The listing builds one solid part. Answer for the finished solid, in the listing's coordinates (mm). A direction names the side the tool comes from. Give positions to 0.01 mm unless a question says otherwise; leave off trailing zeros. Loops run counter-clockwise (first coordinate to the right, second up) from the corner with the lowest first, then second, coordinate; pieces in that order, holes last. Notation, with made-up numbers: M 77,-25.75 L 122,-25.75 A22 cw 122,-15.75 Z; hole C 86.25,50 d10. An arc over 180 degrees is marked long. One line per item, written item: value. Start each with the question number.
Q1. For faces 1 (the flat face through (-2, -1.4, 1.3)), 2 (the conical face through (-0.09, -1.44, 2.52)), determine the directions among +Z, -Z, +X, -X, +Y, -Y from which every point of the face is accessible in a straight line to the end or side of a thin tool.
Q2. A cutting plane is placed at A-A, the plane x = -11.5. Determine the outline of the cut face in (y, z), and give its area (3 significant figures).
Q3. Consider L1, parallel to X at y = 0.5, z = -2.3; L2, parallel to Y at x = -5, z = -0.6; L3, parallel to Y at x = -13, z = -0.8. Determine where each line is inside the solid, lowest interval first.
Q4. Flat-ended cylindrical pins translate along their axes: pin 1 (1.5 mm diameter, centred on x = -29.5, y = 2, fed in from -Z); pin 2 (2 mm diameter, centred on x = -9.5, z = 1.5, fed in from -Y); pin 3 (1.6 mm diameter, centred on y = -1, z = 0.5, fed in from -X); pin 4 (1 mm diameter, centred on y = -1, z = 2, fed in from -X). Find the tip coordinate at first contact, or state that the pin passes through.
from build123d import *

# Parameters (mm, degrees)
DODANIE_WYCI_GNI_CIE1_DEPTH = 2
SFAZOWANIE1_SIZE            = 0.5


with BuildPart() as part:
    # Szkic1 → Obrót1 (revolve)
    with BuildSketch(Plane.XY):
        Polygon((0, 0), (0, 2.75), (-2, 2.75), (-2, 1.5), (-37, 1.5), (-37, 0), align=None)
    revolve(axis=Axis((-37, 0, 0), (1, 0, 0)))

    # Szkic2 → Dodanie-wyciągnięcie1 (add)
    with BuildSketch(Plane(origin=(0, 0, 0), x_dir=(0, 0, -1), z_dir=(1, 0, 0))):
        Polygon((-2.75, 1.58771324), (-2.75, -1.58771324), (0, -3.175426481), (2.75, -1.58771324), (2.75, 1.58771324), (0, 3.175426481), align=None)
    extrude(amount=-DODANIE_WYCI_GNI_CIE1_DEPTH)

    # Sfazowanie1
    sfazowanie1_edges = [part.edges().sort_by_distance(p)[0] for p in [
        (-37, -1.5, 0),
    ]]
    chamfer(sfazowanie1_edges, length=SFAZOWANIE1_SIZE)

    # Szkic9 → Wycięcie-obrót1 (revolve, cut)
    with BuildSketch(Plane.XY):
        Polygon((0, 3.175426481), (0, 2.75), (-0.245620093, 3.175426481), align=None)
    revolve(axis=Axis((-37, 0, 0), (1, 0, 0)), mode=Mode.SUBTRACT)


solid = part.part
Answer block:
1. face 1: -X
1. face 2: +Z, +X, -Y
2. outline: C 0,0 d3
2. area: 7.07 mm^2
3. L1: -2 to 0
3. L2: -1.37 to 1.37
3. L3: -1.27 to 1.27
4. pin 1: z = -0.83
4. pin 2: y = -1.41
4. pin 3: x = -37
4. pin 4: x = -2
